Geometry: final body of the model. Coordinates: model frame, mm. Give positions to 0.01 mm unless a question says otherwise; leave off trailing zeros. Write each loop counter-clockwise with the first axis right and the second up, starting at its lowest first coordinate (ties: lowest second). Pieces come first, ordered by that corner, then holes. Notation, with made-up numbers: (40, -7) -> (46, -7) arc R17 cw to (46, -1) -> close; hole circle Ø11 at (4, 36.25). An arc over 180 degrees is marked (long way). Answer in a Markdown table with one row per item. Add a question column.
Item 1: Section query C-C on z = 1.7. State how many separate pieces and enclosed holes the cut face has, plus the area to 3 significant figures.
Item 2: Material intervals for probe 1 along X at (y, z) = (91, 0.1); probe 2 along Y at (x, z) = (34.5, 1.85); probe 3 along X at (y, z) = (82.5, 0.3), sorted ascending. Write a range as from..to.
Item 3: Section query B-B on y = 40.5. Output: boundary loops of the cut face in (x, z), plus the area to 3 significant figures.
Item 4: Section query A-A on x = 61.5. Output: boundary loops of the cut face in (y, z), plus the area to 3 significant figures.
Item 5: First-contact query: P1, Ø10, axis at x = 18, y = 187.5, coming from the +Z side. Flat tip, straight axial feed; report the tip coordinate or a pass-through.
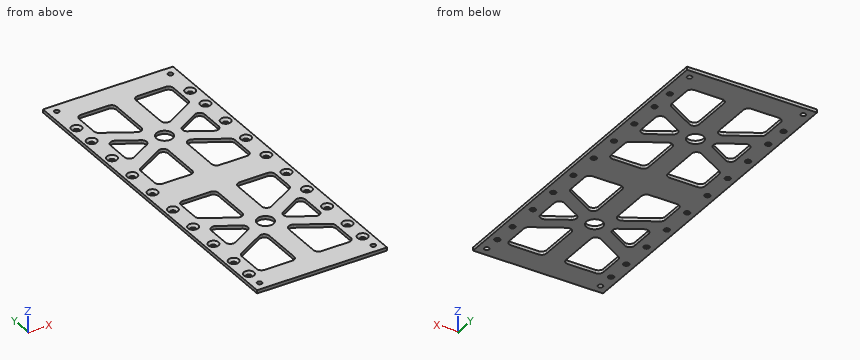
```python
from build123d import *

# Parameters (mm, degrees)
SKETCH1_W                                       = 88
SKETCH1_H                                       = 211
BOSS_EXTRUDE1_DEPTH                             = 2
CUT_EXTRUDE2_DEPTH                              = 2
SKETCH4_R                                       = 5
CUT_EXTRUDE3_DEPTH                              = 3
FILLET2_R                                       = 3
SKETCH5_R                                       = 1.5
CUT_EXTRUDE4_DEPTH                              = 3
SKETCH23_W                                      = 2
SKETCH23_H                                      = 211
SKETCH23_W_2                                    = 2.150374681
CUT_EXTRUDE5_DEPTH                              = 10
SKETCH29_W                                      = 5.911493913
SKETCH29_H                                      = 211
SKETCH29_W_2                                    = 4.036537762
CUT_EXTRUDE10_DEPTH                             = 2
CSK_FOR_M3_FLAT_HEAD_MACHINE_SCREW1_D           = 3.4
CSK_FOR_M3_FLAT_HEAD_MACHINE_SCREW1_DEPTH       = 10
CSK_FOR_M3_FLAT_HEAD_MACHINE_SCREW1_CSINK_D     = 6.3
CSK_FOR_M3_FLAT_HEAD_MACHINE_SCREW1_CSINK_ANGLE = 90
CSK_FOR_M3_FLAT_HEAD_MACHINE_SCREW1_TIP         = 1.021463052


with BuildPart() as part:
    # Sketch1 → Boss-Extrude1 (new body)
    with BuildSketch(Plane.XY):
        with Locations((44, 105.5)):
            Rectangle(SKETCH1_W, SKETCH1_H)
    extrude(amount=BOSS_EXTRUDE1_DEPTH)

    # Sketch3 → Cut-Extrude2 (cut)
    with BuildSketch(Plane.XY.offset(2)):
        Polygon((73, 133.88804004), (50, 147.167096231), (50, 115.5), (73, 115.5), align=None)
        Polygon((38, 115.5), (38, 147.167096231), (15, 133.88804004), (15, 115.5), align=None)
        Polygon((15, 143.125644347), (36, 155.25), (15, 167.374355653), align=None)
        Polygon((73, 143.125644347), (73, 167.374355653), (52, 155.25), align=None)
        Polygon((73, 196), (50, 196), (50, 163.332903769), (73, 176.61195996), align=None)
        Polygon((38, 163.332903769), (38, 196), (15, 196), (15, 176.61195996), align=None)
    cut_extrude2 = extrude(amount=-CUT_EXTRUDE2_DEPTH, mode=Mode.SUBTRACT)

    # Sketch4 → Cut-Extrude3 (cut, through all)
    with BuildSketch(Plane.XY.offset(2)):
        with Locations((44, 155.25)):
            Circle(SKETCH4_R)
    cut_extrude3 = extrude(amount=-CUT_EXTRUDE3_DEPTH, mode=Mode.SUBTRACT)

    # Mirror2: Cut-Extrude2, Cut-Extrude3 across plane
    add(cut_extrude2.mirror(Plane.ZX.offset(105.5)), mode=Mode.SUBTRACT)
    add(cut_extrude3.mirror(Plane.ZX.offset(105.5)), mode=Mode.SUBTRACT)

    # Fillet2
    fillet2_edges = [part.edges().sort_by_distance(p)[0] for p in [
        (36, 55.75, 1),
        (15, 43.625644347, 1),
        (15, 67.874355653, 1),
        (38, 95.5, 1),
        (38, 63.832903769, 1),
        (15, 77.11195996, 1),
        (15, 95.5, 1),
        (73, 15, 1),
        (50, 15, 1),
        (50, 47.667096231, 1),
        (73, 34.38804004, 1),
        (73, 43.625644347, 1),
        (52, 55.75, 1),
        (73, 67.874355653, 1),
        (15, 15, 1),
        (15, 34.38804004, 1),
        (38, 47.667096231, 1),
        (38, 15, 1),
        (73, 77.11195996, 1),
        (50, 63.832903769, 1),
        (50, 95.5, 1),
        (73, 95.5, 1),
        (15, 167.374355653, 1),
        (36, 155.25, 1),
        (15, 143.125644347, 1),
        (38, 147.167096231, 1),
        (38, 115.5, 1),
        (15, 115.5, 1),
        (15, 133.88804004, 1),
        (50, 196, 1),
        (73, 196, 1),
        (73, 176.61195996, 1),
        (50, 163.332903769, 1),
        (52, 155.25, 1),
        (73, 167.374355653, 1),
        (73, 143.125644347, 1),
        (15, 176.61195996, 1),
        (15, 196, 1),
        (38, 196, 1),
        (38, 163.332903769, 1),
        (50, 147.167096231, 1),
        (73, 133.88804004, 1),
        (73, 115.5, 1),
        (50, 115.5, 1),
    ]]
    fillet(fillet2_edges, radius=FILLET2_R)

    # Sketch5 → Cut-Extrude4 (cut, through all)
    with BuildSketch(Plane.XY.offset(2)):
        with Locations((9, 205.5)):
            Circle(SKETCH5_R)
        with Locations((79, 205.5)):
            Circle(SKETCH5_R)
        with Locations((9, 5.5)):
            Circle(SKETCH5_R)
        with Locations((79, 5.5)):
            Circle(SKETCH5_R)
    extrude(amount=-CUT_EXTRUDE4_DEPTH, mode=Mode.SUBTRACT)

    # Sketch23 → Cut-Extrude5 (cut)
    with BuildSketch(Plane.XY.offset(2)):
        with Locations((87, 105.5)):
            Rectangle(SKETCH23_W, SKETCH23_H)
        with Locations((1.075187341, 105.5)):
            Rectangle(SKETCH23_W_2, SKETCH23_H)
    extrude(amount=-CUT_EXTRUDE5_DEPTH, mode=Mode.SUBTRACT)

    # Sketch29 → Cut-Extrude10 (cut)
    with BuildSketch(Plane(origin=(0, 0, 0), x_dir=(-1, 0, 0), z_dir=(0, 0, -1))):
        with Locations((-1.044253043, 105.5)):
            Rectangle(SKETCH29_W, SKETCH29_H)
        with Locations((-86.018268881, 105.5)):
            Rectangle(SKETCH29_W_2, SKETCH29_H)
    extrude(amount=-CUT_EXTRUDE10_DEPTH, mode=Mode.SUBTRACT)

    # CSK for M3 Flat Head Machine Screw1
    with Locations(Plane.XY.offset(2)):
        with Locations((9, 186), (9, 171), (9, 151), (9, 131), (9, 111), (9, 91), (9, 71), (9, 51), (9, 31), (9, 16), (79, 186), (79, 171), (79, 151), (79, 131), (79, 111), (79, 91), (79, 71), (79, 51), (79, 31), (79, 16)):
            CounterSinkHole(CSK_FOR_M3_FLAT_HEAD_MACHINE_SCREW1_D / 2, CSK_FOR_M3_FLAT_HEAD_MACHINE_SCREW1_CSINK_D / 2, depth=CSK_FOR_M3_FLAT_HEAD_MACHINE_SCREW1_DEPTH, counter_sink_angle=CSK_FOR_M3_FLAT_HEAD_MACHINE_SCREW1_CSINK_ANGLE)
            with Locations((0, 0, -(CSK_FOR_M3_FLAT_HEAD_MACHINE_SCREW1_DEPTH + CSK_FOR_M3_FLAT_HEAD_MACHINE_SCREW1_TIP / 2))):  # 118° drill point
                Cone(0, CSK_FOR_M3_FLAT_HEAD_MACHINE_SCREW1_D / 2, CSK_FOR_M3_FLAT_HEAD_MACHINE_SCREW1_TIP, mode=Mode.SUBTRACT)


solid = part.part
```
Findings below:
| question | item | result |
|---|---|---|
| 1 | separate pieces | 1 |
| 1 | enclosed holes | 38 |
| 1 | area | 10,600 mm^2 |
| 2 | probe 1 | x = 4..7.3, 10.7..15, 38..50, 73..77.3, 80.7..84 |
| 2 | probe 2 | y = 0..15, 45.43..66.07, 95.5..115.5, 144.93..165.57, 196..211 |
| 2 | probe 3 | x = 4..15, 38..50, 73..84 |
| 3 | outline | (4, 0) -> (25.59, 0) -> (25.59, 2) -> (4, 2) -> close; (38, 0) -> (50, 0) -> (50, 2) -> (38, 2) -> close; (62.41, 0) -> (84, 0) -> (84, 2) -> (62.41, 2) -> close |
| 3 | area | 110 mm^2 |
| 4 | outline | (0, 0) -> (15, 0) -> (15, 2) -> (0, 2) -> close; (41.03, 0) -> (50.27, 0) -> (50.27, 2) -> (41.03, 2) -> close; (61.23, 0) -> (70.47, 0) -> (70.47, 2) -> (61.23, 2) -> close; (95.5, 0) -> (115.5, 0) -> (115.5, 2) -> (95.5, 2) -> close; (140.53, 0) -> (149.77, 0) -> (149.77, 2) -> (140.53, 2) -> close; (160.73, 0) -> (169.97, 0) -> (169.97, 2) -> (160.73, 2) -> close; (196, 0) -> (211, 0) -> (211, 2) -> (196, 2) -> close |
| 4 | area | 174 mm^2 |
| 5 | P1 | stops at z = 2 |
